Geometry check sheet. Reference: the model listing, model coordinates, mm. A direction names the side the tool comes from. Round coordinates to 2 decimals unless told otherwise and drop trailing zeros. Write each loop counter-clockwise with the first axis right and the second up, starting at its lowest first coordinate (ties: lowest second). Pieces come first, ordered by that corner, then holes. Notation, with made-up numbers: (-10, 50.5) -> (22, 50.5) arc R28 cw to (22, 68.5) -> close; hole circle Ø7 at (6, -37.75). An arc over 180 degrees is marked (long way). Put each result on its own line as item: value. Start each with the question number.
from build123d import *

# Parameters (mm, degrees)
F1_DEPTH = 18
F2_W     = 16
F2_H     = 4
F3_DEPTH = 400
F5_D     = 6
F5_DEPTH = 8
F5_TIP   = 1.8025818571
F7_D     = 6.1
F7_DEPTH = 8
F7_TIP   = 1.832624888


with BuildPart() as f1:
    # F0 (on Front) → F1 (new body)
    with BuildSketch(Plane.XZ):
        with BuildLine():
            ThreePointArc((-397.8999233717, -7.1662084662), (-401.4354572777, -8.6306745602), (-402.8999233717, -12.1662084662))
            Line((-402.8999233717, -12.1662084662), (-402.8999233717, -24.1662084662))
            Line((-402.8999233717, -24.1662084662), (-4.8999233717, -24.1662084662))
            Line((-4.8999233717, -24.1662084662), (-4.8999233717, 15.8337915338))
            Line((-4.8999233717, 15.8337915338), (-121.3999233717, 15.8337915338))
            Line((-121.3999233717, 15.8337915338), (-121.3999233717, 1.8337915338))
            ThreePointArc((-121.3999233717, 1.8337915338), (-122.8643894658, -1.7017423721), (-126.3999233717, -3.1662084662))
            Line((-126.3999233717, -3.1662084662), (-131.3999233717, -3.1662084662))
            ThreePointArc((-131.3999233717, -3.1662084662), (-134.9354572777, -1.7017423721), (-136.3999233717, 1.8337915338))
            Line((-136.3999233717, 1.8337915338), (-136.3999233717, 15.8337915338))
            Line((-136.3999233717, 15.8337915338), (-382.8999233717, 15.8337915338))
            ThreePointArc((-382.8999233717, 15.8337915338), (-386.4354572777, 14.3693254398), (-387.8999233717, 10.8337915338))
            Line((-387.8999233717, 10.8337915338), (-387.8999233717, -2.1662084662))
            ThreePointArc((-387.8999233717, -2.1662084662), (-389.3643894658, -5.7017423721), (-392.8999233717, -7.1662084662))
            Line((-392.8999233717, -7.1662084662), (-397.8999233717, -7.1662084662))
        make_face()
        with BuildLine():
            ThreePointArc((-330.8999233717, 2.8337915338), (-325.8999233717, -2.1662084662), (-330.8999233717, -7.1662084662))
            Line((-330.8999233717, -7.1662084662), (-360.8999233717, -7.1662084662))
            ThreePointArc((-360.8999233717, -7.1662084662), (-365.8999233717, -2.1662084662), (-360.8999233717, 2.8337915338))
            Line((-360.8999233717, 2.8337915338), (-330.8999233717, 2.8337915338))
        make_face(mode=Mode.SUBTRACT)
        with BuildLine():
            ThreePointArc((-268.8999233717, 2.8337915338), (-263.8999233717, -2.1662084662), (-268.8999233717, -7.1662084662))
            Line((-268.8999233717, -7.1662084662), (-298.8999233717, -7.1662084662))
            ThreePointArc((-298.8999233717, -7.1662084662), (-303.8999233717, -2.1662084662), (-298.8999233717, 2.8337915338))
            Line((-298.8999233717, 2.8337915338), (-268.8999233717, 2.8337915338))
        make_face(mode=Mode.SUBTRACT)
        with BuildLine():
            ThreePointArc((-206.8999233717, 2.8337915338), (-201.8999233717, -2.1662084662), (-206.8999233717, -7.1662084662))
            Line((-206.8999233717, -7.1662084662), (-236.8999233717, -7.1662084662))
            ThreePointArc((-236.8999233717, -7.1662084662), (-241.8999233717, -2.1662084662), (-236.8999233717, 2.8337915338))
            Line((-236.8999233717, 2.8337915338), (-206.8999233717, 2.8337915338))
        make_face(mode=Mode.SUBTRACT)
        with BuildLine():
            ThreePointArc((-144.8999233717, 2.8337915338), (-139.8999233717, -2.1662084662), (-144.8999233717, -7.1662084662))
            Line((-144.8999233717, -7.1662084662), (-174.8999233717, -7.1662084662))
            ThreePointArc((-174.8999233717, -7.1662084662), (-179.8999233717, -2.1662084662), (-174.8999233717, 2.8337915338))
            Line((-174.8999233717, 2.8337915338), (-144.8999233717, 2.8337915338))
        make_face(mode=Mode.SUBTRACT)
        with BuildLine():
            ThreePointArc((-82.8999233717, 2.8337915338), (-77.8999233717, -2.1662084662), (-82.8999233717, -7.1662084662))
            Line((-82.8999233717, -7.1662084662), (-112.8999233717, -7.1662084662))
            ThreePointArc((-112.8999233717, -7.1662084662), (-117.8999233717, -2.1662084662), (-112.8999233717, 2.8337915338))
            Line((-112.8999233717, 2.8337915338), (-82.8999233717, 2.8337915338))
        make_face(mode=Mode.SUBTRACT)
        with BuildLine():
            ThreePointArc((-20.8999233717, 2.8337915338), (-15.8999233717, -2.1662084662), (-20.8999233717, -7.1662084662))
            Line((-20.8999233717, -7.1662084662), (-50.8999233717, -7.1662084662))
            ThreePointArc((-50.8999233717, -7.1662084662), (-55.8999233717, -2.1662084662), (-50.8999233717, 2.8337915338))
            Line((-50.8999233717, 2.8337915338), (-20.8999233717, 2.8337915338))
        make_face(mode=Mode.SUBTRACT)
    extrude(amount=F1_DEPTH)

    # F2 (on face) → F3 (cut)
    with BuildSketch(Plane(origin=(-402.8999233717, 0, 0), x_dir=(0, -1, 0), z_dir=(-1, 0, 0))):
        with Locations((8, -22.1662084662)):
            Rectangle(F2_W, F2_H)
    extrude(amount=-F3_DEPTH, mode=Mode.SUBTRACT)

    # F5
    with Locations(Plane(origin=(0, 0, -20.1662084662), x_dir=(1, 0, 0), z_dir=(0, 0, -1))):
        with Locations((-302.8999233717, 11), (-122.8999233717, 11)):
            Hole(F5_D / 2, depth=F5_DEPTH)
            with Locations((0, 0, -(F5_DEPTH + F5_TIP / 2))):  # 118° drill point
                Cone(0, F5_D / 2, F5_TIP, mode=Mode.SUBTRACT)

    # F7
    with Locations(Plane(origin=(0, 0, 0), x_dir=(-1, 0, 0), z_dir=(0, 1, 0))):
        with Locations((392.8999233717, -15.6662084662)):
            Hole(F7_D / 2, depth=F7_DEPTH)
            with Locations((0, 0, -(F7_DEPTH + F7_TIP / 2))):  # 118° drill point
                Cone(0, F7_D / 2, F7_TIP, mode=Mode.SUBTRACT)


solid = f1.part
(1) Sectioned sample at A-A (x = -252.5). Record the cut outline in (y, z), and give its area (3 significant figures).
(2) Set-up check for faces 4 (the flat face through (-98, -9, -7.166)), 5 (the flat face through (-121.4, -9, 9)), 6 (the conical face through (-392.371, -9.514, -15.643)): record each of +Z, -Z, +X, -X, +Y, -Y from which the full face is reachable in a straight line by a thin tool's end or side.
(3) Sectioned sample at B-B (y = -4). State how many separate pieces and enclosed holes the cut face has, and give its area (3 significant figures).
(4) Material ranges on L1, parallel to Z at x = -147, y = -1.75; L2, parallel to X at y = -5, z = 8; L3, parallel to X at y = -1.75, z = -15, recorded low to high. Write a range as from..to.
(5) Mould release check, pull along X, two halves, no side actions. Record for faces 1 (the flat face through (-387.9, -9, 4)), 2 (the cylindrical face through (-139.9, -8.9, -2.1)), 3 (the flat face through (-207, -18, -8)): +X half, -X half, draft (parallel to the pull), parting line (faces both ways), or undercut.
(6) Go/stop test with flat-tipped pins: pin 1 Ø1 at (x, y) = (-310, -3.5) entering from -Z; pin 2 Ø2 at (x, z) = (-150, -22.5) entering from +Y; pin 3 Ø1.5 at (x, z) = (-210, 1) entering from -Y; pin 4 Ø1.5 at (x, y) = (-129, -11) entering from +Z. Record where each tip stops, or that it passes through.
Found:
1. outline: (-18, -24.17) -> (-16, -24.17) -> (-16, -20.17) -> (0, -20.17) -> (0, 15.83) -> (-18, 15.83) -> close
1. area: 656 mm2
2. face 4: +Y, -Y
2. face 5: +Z, +Y, -Y
2. face 6: +Y
3. separate pieces: 1
3. enclosed holes: 7
3. area: 11,400 mm2
4. L1: -20.17..-7.17, 2.83..15.83
4. L2: -387.9..-136.4, -121.4..-4.9
4. L3: -402.9..-395.88, -389.92..-4.9
5. face 1: -X half
5. face 2: undercut
5. face 3: draft
6. pin 1: z = -20.17
6. pin 2: y = -16
6. pin 3: through
6. pin 4: z = -3.17
